Work out the finished part from the listing and answer in its coordinate system (mm). A direction names the side the tool comes from. Give positions to 0.01 mm unless a question says otherwise; leave off trailing zeros. Write each loop counter-clockwise with the first axis right and the second up, starting at its lowest first coordinate (ties: lowest second). Pieces come first, ordered by that corner, then holes. Notation, with made-up numbers: (66, 78) -> (116, 78) arc R22 ccw to (116, 116) -> close; hole circle Ø3 at (32, 10.5). An arc over 180 degrees is marked (long way). Write item = value, one per line. Start each with the question number.
from build123d import *

# Parameters (mm, degrees)
SKETCH1_R           = 14
BOSS_EXTRUDE1_DEPTH = 3
SKETCH2_R           = 6.2
CUT_EXTRUDE1_DEPTH  = 8
BOSS_EXTRUDE2_START = 35
SKETCH3_R           = 14
SKETCH3_R_2         = 11.5
BOSS_EXTRUDE2_DEPTH = 35
CUT_EXTRUDE2_DEPTH  = 63.617888818


with BuildPart() as part:
    # Sketch1 → Boss-Extrude1 (new body)
    with BuildSketch(Plane.XY):
        with Locations((22.5, 0)):
            Circle(SKETCH1_R)
        with BuildLine():
            Line((0, 5), (45, 5))
            ThreePointArc((45, 5), (50, 0), (45, -5))
            Line((45, -5), (0, -5))
            ThreePointArc((0, -5), (-5, 0), (0, 5))
        make_face()
    extrude(amount=BOSS_EXTRUDE1_DEPTH)

    # Sketch2 → Cut-Extrude1 (cut)
    with BuildSketch(Plane(origin=(0, 0, 0), x_dir=(-1, 0, 0), z_dir=(0, 0, -1))):
        with Locations((-22.5, 0)):
            Circle(SKETCH2_R)
    extrude(amount=-CUT_EXTRUDE1_DEPTH, mode=Mode.SUBTRACT)

    # Sketch3 → Boss-Extrude2 (add)
    with BuildSketch(Plane(origin=(0, 0, 0), x_dir=(-1, 0, 0), z_dir=(0, 0, -1)).offset(BOSS_EXTRUDE2_START)):
        with Locations((-22.5, 0)):
            Circle(SKETCH3_R)
        with Locations((-22.5, 0)):
            Circle(SKETCH3_R_2, mode=Mode.SUBTRACT)
    extrude(amount=-BOSS_EXTRUDE2_DEPTH)

    # Sketch4 → Cut-Extrude2 (cut, through all)
    with BuildSketch(Plane(origin=(0, 0, 0), x_dir=(-1, 0, 0), z_dir=(0, 0, -1))):
        with BuildLine():
            Line((-40, -2.5), (-45, -2.5))
            ThreePointArc((-45, -2.5), (-47.5, 0), (-45, 2.5))
            Line((-45, 2.5), (-40, 2.5))
            ThreePointArc((-40, 2.5), (-37.5, 0), (-40, -2.5))
        make_face()
        with BuildLine():
            Line((-5, 2.5), (0, 2.5))
            ThreePointArc((0, 2.5), (2.5, 0), (0, -2.5))
            Line((0, -2.5), (-5, -2.5))
            ThreePointArc((-5, -2.5), (-7.5, 0), (-5, 2.5))
        make_face()
    extrude(amount=-CUT_EXTRUDE2_DEPTH, mode=Mode.SUBTRACT)


solid = part.part
(1) A cutting plane is placed at B-B, the plane y = 0. Write down the section's boundary in (x, z).
(2) A cutting plane is placed at D-D, the plane z = -20.5. Write down the section's boundary in (x, y).
(3) Each of these flat-tipped pins is pushed along its axis until it touches: pin 1 (1.5 mm diameter, centred on x = 42, z = 1.5, fed in from +Y); pin 2 (3.5 mm diameter, centred on x = 41.5, z = 1, fed in from -Y); pin 3 (2 mm diameter, centred on x = 11.5, z = -12.5, fed in from +Y). Where does it stop, or does it pass through?
(4) A cutting plane is placed at C-C, the plane y = 4.25. Write down the section's boundary in (x, z), then the cut area to 3 significant figures.
(5) Determine the mould class of faces 1 (the flat face through (28.2, -2.9, 3)), 2 (the flat face through (43, 2.5, 1)), 3 (the cylindrical face through (50, 0, 1)) for opening direction X: pulls with the +X half, pulls with the -X half, needs draft (parallel to the pull), parting line crosses it, or undercut.
(6) A cutting plane is placed at A-A, the plane x = 22.5. Write down the section's boundary in (y, z).
(7) For faces 4 (the flat face through (5, -5, 1)), 5 (the flat face through (40, 5, 1)), 6 (the cylindrical face through (7.5, -0.1, 1.5)), 7 (the cylindrical face through (11.53, 3.45, -17.74)), determine the directions among +Z, -Z, +X, -X, +Y, -Y from which every point of the face is accessible in a straight line to the end or side of a thin tool.
(8) Find the intervals of material crossed by line 1 along Y through (x, z) = (22.5, 2); line 2 along Y through (x, z) = (22.5, -12); line 3 along Z through (x, y) = (24, -9.25), in increasing order.
Results list:
q1.outline = (-5, 0) -> (-2.5, 0) -> (-2.5, 3) -> (-5, 3) -> close; (7.5, 0) -> (8.5, 0) -> (8.5, -35) -> (11, -35) -> (11, 0) -> (16.3, 0) -> (16.3, 3) -> (7.5, 3) -> close; (28.7, 0) -> (34, 0) -> (34, -35) -> (36.5, -35) -> (36.5, 0) -> (37.5, 0) -> (37.5, 3) -> (28.7, 3) -> close; (47.5, 0) -> (50, 0) -> (50, 3) -> (47.5, 3) -> close
q2.outline = circle Ø28 at (22.5, 0); hole circle Ø23 at (22.5, 0)
q3.pin_1 = 5
q3.pin_2 = -5
q3.pin_3 = 9.8
q4.outline = (-2.63, 0) -> (9.16, 0) -> (9.16, -35) -> (11.81, -35) -> (11.81, 0) -> (17.99, 0) -> (17.99, 3) -> (-2.63, 3) -> close; (27.01, 0) -> (33.19, 0) -> (33.19, -35) -> (35.84, -35) -> (35.84, 0) -> (47.63, 0) -> (47.63, 3) -> (27.01, 3) -> close
q4.area = 309 mm²
q5.face_1 = needs draft
q5.face_2 = undercut
q5.face_3 = pulls with the +X half
q6.outline = (-14, -35) -> (-11.5, -35) -> (-11.5, 0) -> (-6.2, 0) -> (-6.2, 3) -> (-14, 3) -> close; (6.2, 0) -> (11.5, 0) -> (11.5, -35) -> (14, -35) -> (14, 3) -> (6.2, 3) -> close
q7.face_4 = +Z, -Z, -X, -Y
q7.face_5 = +Z, -Z, +X, +Y
q7.face_6 = +Z, -Z
q7.face_7 = -Z
q8.line_1 = -14 to -6.2, 6.2 to 14
q8.line_2 = -14 to -11.5, 11.5 to 14
q8.line_3 = 0 to 3
